CAD build for the part. Positions are in the model's coordinates, mm. A direction names the side the tool comes from. Give positions to 0.01 mm unless a question says otherwise; leave off trailing zeros. Write each loop counter-clockwise with the first axis right and the second up, starting at its lowest first coordinate (ties: lowest second). Pieces come first, ordered by that corner, then holes. Notation, with made-up numbers: (63.25, -33) - (107.25, -33) arc R22 cw to (107.25, -26) - close; hole circle Ø9 at (32.5, 42). An arc over 180 degrees is marked (long way). Answer as a JSON object with one key per item and string values.
from build123d import *

# Parameters (mm, degrees)
F0_W      = 355.6
F0_H      = 76.2
F0_R      = 10.3505
F0_R_2    = 13.716
F1_DEPTH  = 37.084
F2_R      = 6.35
F3_W      = 304.8
F3_H      = 12.7
F3_R      = 10.3505
F3_R_2    = 13.716
F4_DEPTH  = 2.54
F5_R      = 10.3505
F5_R_2    = 13.716
F6_DEPTH  = 2.54
F8_DEPTH  = 304.8
F10_DEPTH = 304.8


with BuildPart() as f1:
    # F0 (on Top) → F1 (new body)
    with BuildSketch(Plane.XY):
        Rectangle(F0_W, F0_H)
        with Locations((-100.076, 0)):
            Circle(F0_R, mode=Mode.SUBTRACT)
        Circle(F0_R_2, mode=Mode.SUBTRACT)
        with Locations((100.076, 0)):
            Circle(F0_R, mode=Mode.SUBTRACT)
    extrude(amount=F1_DEPTH)

    # F2
    f2_edges = [f1.edges().sort_by_distance(p)[0] for p in [
        (0, -38.1, 37.084),
        (0, -38.1, 0),
        (0, 38.1, 37.084),
        (0, 38.1, 0),
    ]]
    fillet(f2_edges, radius=F2_R)

    # F3 (on face) → F4 (join)
    with BuildSketch(Plane.XY.offset(37.084)):
        with Locations((0, -38.1)):
            Rectangle(F3_W, F3_H)
        Polygon((-152.4, -12.7), (-152.4, -31.75), (152.4, -31.75), (152.4, -12.7), (133.35, 25.4), (-133.35, 25.4), align=None)
        with Locations((-100.076, 0)):
            Circle(F3_R, mode=Mode.SUBTRACT)
        Circle(F3_R_2, mode=Mode.SUBTRACT)
        with Locations((100.076, 0)):
            Circle(F3_R, mode=Mode.SUBTRACT)
    extrude(amount=F4_DEPTH)

    # F5 (on face) → F6 (join)
    with BuildSketch(Plane(origin=(0, 0, 0), x_dir=(1, 0, 0), z_dir=(0, 0, -1))):
        Polygon((-152.4, 12.7), (-133.35, -25.4), (133.35, -25.4), (152.4, 12.7), (152.4, 31.75), (-152.4, 31.75), align=None)
        with Locations((-100.076, 0)):
            Circle(F5_R, mode=Mode.SUBTRACT)
        Circle(F5_R_2, mode=Mode.SUBTRACT)
        with Locations((100.076, 0)):
            Circle(F5_R, mode=Mode.SUBTRACT)
    extrude(amount=F6_DEPTH)

    # F7 (on face) → F8 (join)
    with BuildSketch(Plane.YZ.offset(152.4)):
        with BuildLine():
            ThreePointArc((-48.26, 33.274), (-47.1440768363, 35.9680768363), (-44.45, 37.084))
            Line((-44.45, 37.084), (-44.45, 39.624))
            ThreePointArc((-44.45, 39.624), (-48.9401280605, 37.7641280605), (-50.8, 33.274))
            Line((-50.8, 33.274), (-50.8, 25.654))
            ThreePointArc((-50.8, 25.654), (-48.9401280605, 21.1638719395), (-44.45, 19.304))
            Line((-44.45, 19.304), (-40.64, 19.304))
            Line((-40.64, 19.304), (-40.64, 21.844))
            Line((-40.64, 21.844), (-44.45, 21.844))
            ThreePointArc((-44.45, 21.844), (-47.1440768363, 22.9599231637), (-48.26, 25.654))
            Line((-48.26, 25.654), (-48.26, 33.274))
        make_face()
    extrude(amount=-F8_DEPTH)

    # F9 (on face) → F10 (join)
    with BuildSketch(Plane(origin=(-152.4, 0, 0), x_dir=(0, -1, 0), z_dir=(-1, 0, 0))):
        with BuildLine():
            ThreePointArc((31.75, -2.54), (38.0361792847, 0.0638207153), (40.64, 6.35))
            Line((40.64, 6.35), (40.64, 12.7))
            Line((40.64, 12.7), (38.1, 12.7))
            Line((38.1, 12.7), (38.1, 6.35))
            ThreePointArc((38.1, 6.35), (36.2401280605, 1.8598719395), (31.75, 0))
            Line((31.75, 0), (31.75, -2.54))
        make_face()
    extrude(amount=-F10_DEPTH)


solid = f1.part
Item 1: Probe line 1 (X direction, y = 0, z = 12); line 2 (Y direction, x = 0, z = 28); line 3 (Y direction, x = -130, z = 25.5). List the from-to ranges inside material, lowest first. Write a range as from..to.
Entries:
{"line 1": "-177.8..-110.43, -89.73..-13.72, 13.72..89.73, 110.43..177.8", "line 2": "-50.8..-48.26, -38.1..-13.72, 13.72..38.1", "line 3": "-50.8..-48.26, -38.1..38.1"}
Item 2: Cut at A-A (y = 0). Give the cut face in (x, z), and give its area (3 significant figures).
Entries:
{"outline": "(-177.8, 0) - (-146.05, 0) - (-146.05, -2.54) - (-110.43, -2.54) - (-110.43, 39.62) - (-146.05, 39.62) - (-146.05, 37.08) - (-177.8, 37.08) - close; (-89.73, -2.54) - (-13.72, -2.54) - (-13.72, 39.62) - (-89.73, 39.62) - close; (13.72, -2.54) - (89.73, -2.54) - (89.73, 39.62) - (13.72, 39.62) - close; (110.43, -2.54) - (146.05, -2.54) - (146.05, 0) - (177.8, 0) - (177.8, 37.08) - (146.05, 37.08) - (146.05, 39.62) - (110.43, 39.62) - close", "area": "11,800 mm2"}
Item 3: Cut at C-C (x = 57). Give the cut face in (y, z), and give its area (3 significant figures).
Entries:
{"outline": "(-50.8, 25.65) arc R6.35 ccw to (-44.45, 19.3) - (-40.64, 19.3) - (-40.64, 21.84) - (-44.45, 21.84) arc R3.81 cw to (-48.26, 25.65) - (-48.26, 33.27) arc R3.81 cw to (-44.45, 37.08) - (-31.75, 37.08) arc R6.35 ccw to (-38.1, 30.73) - (-38.1, 12.7) - (-40.64, 12.7) - (-40.64, 6.35) arc R8.89 ccw to (-31.75, -2.54) - (25.4, -2.54) - (25.4, 0) - (31.75, 0) arc R6.35 ccw to (38.1, 6.35) - (38.1, 30.73) arc R6.35 ccw to (31.75, 37.08) - (25.4, 37.08) - (25.4, 39.62) - (-44.45, 39.62) arc R6.35 ccw to (-50.8, 33.27) - close", "area": "3,230 mm2"}
Item 4: Mould opens along Y. For faces 4 (the flat face through (152.4, -31, -1)), 5 (the cylindrical face through (-2.13, -37.97, 0)), 6 (the flat face through (2, -48.26, 29)) say: +Y half, -Y half, draft (parallel to the pull), parting line (faces both ways), or undercut.
Entries:
{"face 4": "draft", "face 5": "-Y half", "face 6": "undercut"}
Item 5: Cut at D-D (x = -105). Give the cut face in (y, z).
Entries:
{"outline": "(-50.8, 25.65) arc R6.35 ccw to (-44.45, 19.3) - (-40.64, 19.3) - (-40.64, 21.84) - (-44.45, 21.84) arc R3.81 cw to (-48.26, 25.65) - (-48.26, 33.27) arc R3.81 cw to (-44.45, 37.08) - (-31.75, 37.08) arc R6.35 ccw to (-38.1, 30.73) - (-38.1, 12.7) - (-40.64, 12.7) - (-40.64, 6.35) arc R8.89 ccw to (-31.75, -2.54) - (-9.1, -2.54) - (-9.1, 39.62) - (-44.45, 39.62) arc R6.35 ccw to (-50.8, 33.27) - close; (9.1, -2.54) - (25.4, -2.54) - (25.4, 0) - (31.75, 0) arc R6.35 ccw to (38.1, 6.35) - (38.1, 30.73) arc R6.35 ccw to (31.75, 37.08) - (25.4, 37.08) - (25.4, 39.62) - (9.1, 39.62) - close"}
Item 6: Cut at B-B (x = 0). Give the cut face in (y, z), and give its area (3 significant figures).
Entries:
{"outline": "(-50.8, 25.65) arc R6.35 ccw to (-44.45, 19.3) - (-40.64, 19.3) - (-40.64, 21.84) - (-44.45, 21.84) arc R3.81 cw to (-48.26, 25.65) - (-48.26, 33.27) arc R3.81 cw to (-44.45, 37.08) - (-31.75, 37.08) arc R6.35 ccw to (-38.1, 30.73) - (-38.1, 12.7) - (-40.64, 12.7) - (-40.64, 6.35) arc R8.89 ccw to (-31.75, -2.54) - (-13.72, -2.54) - (-13.72, 39.62) - (-44.45, 39.62) arc R6.35 ccw to (-50.8, 33.27) - close; (13.72, -2.54) - (25.4, -2.54) - (25.4, 0) - (31.75, 0) arc R6.35 ccw to (38.1, 6.35) - (38.1, 30.73) arc R6.35 ccw to (31.75, 37.08) - (25.4, 37.08) - (25.4, 39.62) - (13.72, 39.62) - close", "area": "2,070 mm2"}
Item 7: Which spindle directions (+Z, -Z, +X, -X, +Y, -Y) get a long thin tool onto all of the face, cutting with end or side? Do faces 1 (the flat face through (-152.4, -39, 38)), 2 (the flat face through (152.4, -39, 38)), 3 (the flat face through (-1, 28, 37.084)). Say none if no direction does.
Entries:
{"face 1": "+Z, -X, -Y", "face 2": "+Z, +X, -Y", "face 3": "+Z, +Y"}
Item 8: Flat gauge pins, fed straight in: P1, Ø10, axis at x = -89, y = 28.5, coming from the +Z side; P2, Ø7, axis at x = -15.5, z = 10, coming from the -Y side; P3, Ø4, axis at x = -39, y = -43.5, coming from the -Z side; P4, Ø4, axis at x = 135, z = 16.5, coming from the -Y side. Where does each tip first touch, or does it go through?
Entries:
{"P1": "z = 39.62", "P2": "y = -40.64", "P3": "z = 19.3", "P4": "y = -38.1"}
